Design review of the part built by this model. Coordinates are the model's own, in mm. Coordinates: 2 decimals unless noted, no trailing zeros. Write each loop counter-clockwise with the first axis right and the second up, starting at its lowest first coordinate (ties: lowest second). Pieces come first, ordered by that corner, then holes.
Q1. For pin 1 Ø4 at (x, y) = (101.6, -6.35) entering from +Z, flat-tipped, find the tip position at first contact; note if it passes through.
Q2. Take a section at C-C, the plane z = 0.45. Write out the cut boundary in (x, y).
Q3. Take a section at B-B, the plane y = -6.35. Write out the cut boundary in (x, z).
Q4. For L1, parallel to Y at x = 101.6, z = 0.5; L2, parallel to X at y = -5, z = 0.65; L3, parallel to X at y = -3.75, z = 0.4, list the stretches that pass through material, from the lowest coordinate up.
Q5. Take a section at A-A, the plane x = 101.6. Write out the cut boundary in (y, z).
from build123d import *

# Parameters (mm, degrees)
F1_DEPTH = 12.7
F3_D     = 6.7564


with BuildPart() as f1:
    # F0 (on Front) → F1 (new body)
    with BuildSketch(Plane.XZ):
        Polygon((0, 0.79375), (0, 0), (203.2, 0), (203.2, 0.79375), (187.6806, 0.79375), (183.8680549408, 0.79375), (19.3244994099, 0.79375), (15.5119543507, 0.79375), align=None)
    extrude(amount=F1_DEPTH)

    # F3 (through all)
    with Locations(Plane.XY.offset(0.79375)):
        with Locations((101.6, -6.35), (38.4429, -6.35), (164.7444, -6.35)):
            Hole(F3_D / 2)


solid = f1.part
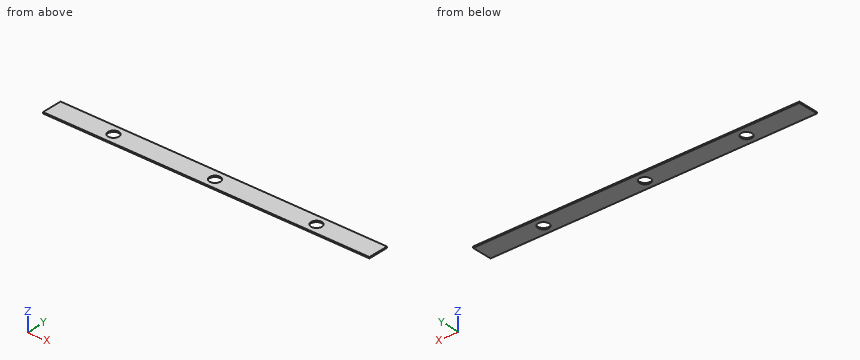
Responses:
1. pin 1: passes through
2. outline: (0, -12.7) - (203.2, -12.7) - (203.2, 0) - (0, 0) - close; hole circle Ø6.76 at (38.44, -6.35); hole circle Ø6.76 at (101.6, -6.35); hole circle Ø6.76 at (164.74, -6.35)
3. outline: (0, 0) - (35.06, 0) - (35.06, 0.79) - (0, 0.79) - close; (41.82, 0) - (98.22, 0) - (98.22, 0.79) - (41.82, 0.79) - close; (104.98, 0) - (161.37, 0) - (161.37, 0.79) - (104.98, 0.79) - close; (168.12, 0) - (203.2, 0) - (203.2, 0.79) - (168.12, 0.79) - close
4. L1: y = -12.7 to -9.73, -2.97 to 0
4. L2: x = 0 to 35.35, 41.54 to 98.5, 104.7 to 161.65, 167.84 to 203.2
4. L3: x = 0 to 36.29, 40.6 to 99.44, 103.76 to 162.59, 166.9 to 203.2
5. outline: (-12.7, 0) - (-9.73, 0) - (-9.73, 0.79) - (-12.7, 0.79) - close; (-2.97, 0) - (0, 0) - (0, 0.79) - (-2.97, 0.79) - close
